Design review of the part built by this model. Coordinates are the model's own, in mm. Round coordinates to 2 decimals unless told otherwise and drop trailing zeros. Write each loop counter-clockwise with the first axis right and the second up, starting at its lowest first coordinate (ties: lowest second). Pieces come first, ordered by that corner, then holes. Notation, with made-up numbers: (-16, 86) -> (14, 86) arc R23 ccw to (14, 117) -> close; hole circle Ø6 at (47, 87). An arc over 180 degrees is marked (long way). One line per question, with ' | ' between items. Start each with the question number.
1) For probe 1 along Y at (x, z) = (200, 1.25); probe 2 along Y at (x, z) = (120, 3.55); probe 3 along Y at (x, z) = (-53.5, 2.2), list the stretches that pass through material, from the lowest coordinate up.
2) Consider section C-C (x = 265). Give the boundary of the cut face in (y, z), then the cut area to 3 significant figures.
3) Consider section A-A (z = 1.4). Give the boundary of the cut face in (x, y).
4) Consider section B-B (y = -41). Give the boundary of the cut face in (x, z).
5) Insertion check: pin 1 Ø5.5 at (x, y) = (0, 0) entering from -Z; pin 2 Ø2 at (x, z) = (75, 3.5) entering from +Y; pin 3 Ø1.5 at (y, z) = (14.5, 1.5) entering from +X. Each pin has a flat end and moves straight along its axis. Give the tip position at first contact, or say it passes through.
```python
from build123d import *

# Parameters (mm, degrees)
SKETCH_1_R      = 3.5
EXTRUDE_1_DEPTH = 5


with BuildPart() as part:
    # 草图1 → 凸台-拉伸1 (new body)
    with BuildSketch(Plane.XY):
        Polygon((-175, 45), (-125, -55), (255, -55), (345, 35), (275, 130), (-115, 140), align=None)
        Circle(SKETCH_1_R, mode=Mode.SUBTRACT)
        with Locations((-80, 60)):
            Circle(SKETCH_1_R, mode=Mode.SUBTRACT)
        with Locations((120, 60)):
            Circle(SKETCH_1_R, mode=Mode.SUBTRACT)
        with Locations((200, -20)):
            Circle(SKETCH_1_R, mode=Mode.SUBTRACT)
        with Locations((-40, 95)):
            Circle(SKETCH_1_R, mode=Mode.SUBTRACT)
        with Locations((135, 95)):
            Circle(SKETCH_1_R, mode=Mode.SUBTRACT)
    extrude(amount=EXTRUDE_1_DEPTH)


solid = part.part
```
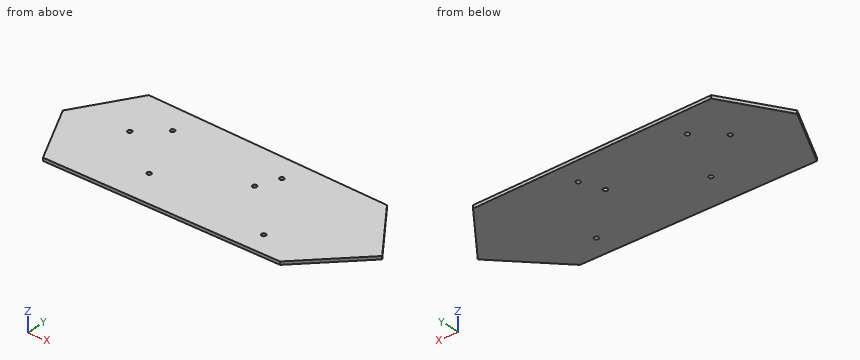
From the geometry:
1) probe 1: y = -55 to -23.5, -16.5 to 131.92 | probe 2: y = -55 to 56.5, 63.5 to 133.97 | probe 3: y = -55 to 138.42
2) outline: (-45, 0) -> (130.26, 0) -> (130.26, 5) -> (-45, 5) -> close | area: 876 mm2
3) outline: (-175, 45) -> (-125, -55) -> (255, -55) -> (345, 35) -> (275, 130) -> (-115, 140) -> close; hole circle Ø7 at (-80, 60); hole circle Ø7 at (-40, 95); hole circle Ø7 at (0, 0); hole circle Ø7 at (120, 60); hole circle Ø7 at (135, 95); hole circle Ø7 at (200, -20)
4) outline: (-132, 0) -> (269, 0) -> (269, 5) -> (-132, 5) -> close
5) pin 1: passes through | pin 2: stops at y = 135.15 | pin 3: stops at x = 325.25
